Read the model definition and answer for the solid it produces. Units are mm, in the model's axes. A direction names the side the tool comes from. Coordinates: 2 decimals unless noted, no trailing zeros. Loops run counter-clockwise (first coordinate to the right, second up) from the corner with the lowest first, then second, coordinate; pieces in that order, holes last. Notation, with made-up numbers: (37.5, 19) - (51.5, 19) arc R34 cw to (51.5, 51) - close; hole circle Ø2 at (-38, 45). An arc over 180 degrees is marked (long way). Use one line per item in the form item = value. Start each with the question number.
1) The mould has two halves that part along Z. Classify faces 1 (the face through (0, -25, -15)), 2 (the face through (14, -25, -3)), 3 (the face through (29, -25, -7)), 4 (the face through (-0.5, -25.4, -8)): released by +Z, released by -Z, zero draft, split by the parting line, or undercut.
2) A cutting plane is placed at B-B (y = -47). Give the vertices of the cut face in (x, z), and give its area (3 significant figures).
3) Which of the six approach directions +Z, -Z, +X, -X, +Y, -Y give full straight-line access (tool end or side, diameter ignored) to faces 5 (the face through (28.5, -25.4, -6)), 6 (the face through (28, -25, -14)), 7 (the face through (31, -25, -11))?
4) A cutting plane is placed at D-D (y = -3.5). Give the vertices of the cut face in (x, z).
5) Each of these flat-tipped pins is pushed along its axis until it touches: P1, Ø3, axis at x = 20.5, y = -44, coming from the -Z side; P2, Ø1.8, axis at x = 14, y = -47, coming from the -Z side. Where does it stop, or does it pass through?
6) A cutting plane is placed at A-A (z = -16). Give the vertices of the cut face in (x, y).
7) Consider line 1 (X direction, y = -47, z = -1.7); line 2 (Y direction, x = 14, z = -0.8); line 3 (X direction, y = -24, z = -15). Determine where each line is inside the solid, lowest interval first.
8) A cutting plane is placed at C-C (x = 14). Give the vertices of the cut face in (y, z), and give its area (3 significant figures).
from build123d import *

# Parameters (mm, degrees)
F0_W           = 28
F0_H           = 3
F1_DEPTH       = 50
F2_W           = 1
F2_H           = 2
F3_DEPTH       = 50
F5_D           = 2
F5_CSINK_D     = 3
F5_CSINK_ANGLE = 90


with BuildPart() as f1:
    # F0 (on Front) → F1 (new body)
    with BuildSketch(Plane.XZ):
        Polygon((0, -3), (0, 0), (-3, 0), (-3, -21), (0, -21), align=None)
        with Locations((14, -1.5)):
            Rectangle(F0_W, F0_H)
        Polygon((31, 0), (28, 0), (28, -3), (28, -21), (31, -21), align=None)
    extrude(amount=F1_DEPTH)

    # F2 (on face) → F3 (cut)
    with BuildSketch(Plane.XZ.offset(50)):
        with Locations((-0.5, -7)):
            Rectangle(F2_W, F2_H)
        with Locations((28.5, -7)):
            Rectangle(F2_W, F2_H)
    extrude(amount=-F3_DEPTH, mode=Mode.SUBTRACT)

    # F5 (through all)
    with Locations(Plane(origin=(0, 0, -3), x_dir=(1, 0, 0), z_dir=(0, 0, -1))):
        with Locations((14, 47)):
            CounterSinkHole(F5_D / 2, F5_CSINK_D / 2, counter_sink_angle=F5_CSINK_ANGLE)


solid = f1.part
Found:
q1.face_1 = zero draft
q1.face_2 = released by -Z
q1.face_3 = undercut
q1.face_4 = undercut
q2.outline = (-3, -21) - (0, -21) - (0, -8) - (-1, -8) - (-1, -6) - (0, -6) - (0, -3) - (12.5, -3) - (13, -2.5) - (13, 0) - (-3, 0) - close; (15, -2.5) - (15.5, -3) - (28, -3) - (28, -6) - (29, -6) - (29, -8) - (28, -8) - (28, -21) - (31, -21) - (31, 0) - (15, 0) - close
q2.area = 200 mm^2
q3.face_5 = +Y, -Y
q3.face_6 = -Z, +Y, -Y
q3.face_7 = +Z, -Z, +X, +Y, -Y
q4.outline = (-3, -21) - (0, -21) - (0, -8) - (-1, -8) - (-1, -6) - (0, -6) - (0, -3) - (28, -3) - (28, -6) - (29, -6) - (29, -8) - (28, -8) - (28, -21) - (31, -21) - (31, 0) - (-3, 0) - close
q5.P1 = -3
q5.P2 = through
q6.outline = (-3, -50) - (0, -50) - (0, 0) - (-3, 0) - close; (28, -50) - (31, -50) - (31, 0) - (28, 0) - close
q7.line_1 = -3 to 13, 15 to 31
q7.line_2 = -50 to -48, -46 to 0
q7.line_3 = -3 to 0, 28 to 31
q8.outline = (-50, -3) - (-48.5, -3) - (-48, -2.5) - (-48, 0) - (-50, 0) - close; (-46, -2.5) - (-45.5, -3) - (0, -3) - (0, 0) - (-46, 0) - close
q8.area = 144 mm^2
